Input: part model. Units: mm. Frame: model coordinates. Face numbers are marked on the shaded views. A direction names the side the tool comes from. Give positions to 0.01 mm unless a question says otherwise; leave off trailing zeros. Loops run counter-clockwise (first coordinate to the right, second up) from the corner with the lowest first, then second, coordinate; pieces in that order, holes last.
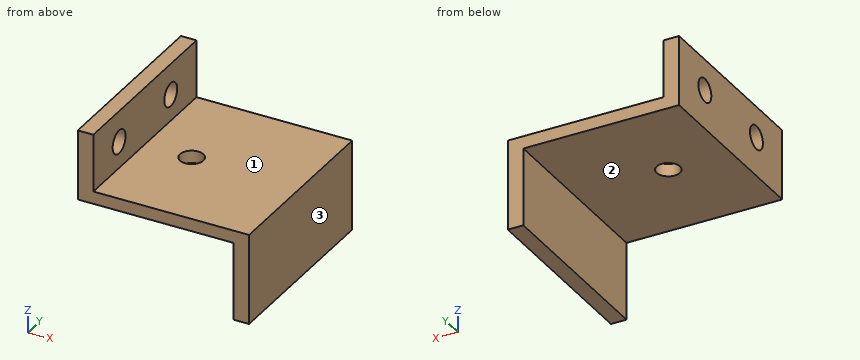
from build123d import *

# Parameters (mm, degrees)
RESSALTO_EXTRUS_O2_DEPTH = 24
ESBO_O2_R                = 1.5
CORTE_EXTRUS_O1_DEPTH    = 24
ESBO_O6_R                = 1.5
CORTE_EXTRUS_O2_DEPTH    = 13


with BuildPart() as part:
    # Esboço1 → Ressalto-extrusão2 (new body)
    with BuildSketch(Plane(origin=(0, 0, 0), x_dir=(1, 0, 0), z_dir=(0, 1, 0))):
        Polygon((0, 0), (0, -7.4), (2, -7.4), (2, 0), (22, 0), (22, 11.6), (20, 11.6), (20, 1.6), (0, 1.6), align=None)
    extrude(amount=RESSALTO_EXTRUS_O2_DEPTH)

    # Esboço2 → Corte-extrusão1 (cut)
    with BuildSketch(Plane.ZY):
        with Locations((3.4, 18)):
            Circle(ESBO_O2_R)
        with Locations((3.4, 6)):
            Circle(ESBO_O2_R)
    extrude(amount=-CORTE_EXTRUS_O1_DEPTH, mode=Mode.SUBTRACT)

    # Esboço6 → Corte-extrusão2 (cut)
    with BuildSketch(Plane(origin=(0, 0, -1.6), x_dir=(-1, 0, 0), z_dir=(0, 0, -1))):
        with Locations((-8, 12)):
            Circle(ESBO_O6_R)
    extrude(amount=-CORTE_EXTRUS_O2_DEPTH, mode=Mode.SUBTRACT)


solid = part.part
(1) Cut plane A-A (y = 12). Return the cut outline in (x, z).
Values follow:
outline: (0, -1.6) - (6.5, -1.6) - (6.5, 0) - (2, 0) - (2, 7.4) - (0, 7.4) - close; (9.5, -1.6) - (20, -1.6) - (20, -11.6) - (22, -11.6) - (22, 0) - (9.5, 0) - close
(2) Pin query (flat end, axial travel): pin 1 Ø2.5 at (x, y) = (8, 12) entering from -Z; pin 2 Ø4 at (x, y) = (17.5, 9) entering from +Z; pin 3 Ø6 at (x, y) = (4.5, 2.5) entering from -Z; pin 4 Ø11 at (y, z) = (10.5, -8.5) entering from -X. Return the tip coordinate at first contact, or that it passes through.
Values follow:
pin 1: passes through
pin 2: stops at z = 0
pin 3: stops at z = -1.6
pin 4: stops at x = 20
(3) Cut plane B-B (z = 3.4). Return the cut outline in (x, y).
Values follow:
outline: (0, 0) - (2, 0) - (2, 4.5) - (0, 4.5) - close; (0, 7.5) - (2, 7.5) - (2, 16.5) - (0, 16.5) - close; (0, 19.5) - (2, 19.5) - (2, 24) - (0, 24) - close
(4) Cut plane D-D (y = 18). Return the cut outline in (x, z), and give its area (3 significant figures).
Values follow:
outline: (0, -1.6) - (20, -1.6) - (20, -11.6) - (22, -11.6) - (22, 0) - (2, 0) - (2, 1.9) - (0, 1.9) - close; (0, 4.9) - (2, 4.9) - (2, 7.4) - (0, 7.4) - close
area: 64.0 mm2
(5) Cut plane C-C (x = 8). Return the cut outline in (y, z), and give its area (3 significant figures).
Values follow:
outline: (0, -1.6) - (10.5, -1.6) - (10.5, 0) - (0, 0) - close; (13.5, -1.6) - (24, -1.6) - (24, 0) - (13.5, 0) - close
area: 33.6 mm2
(6) Ray query, probe 1 along Y at (x, z) = (0.5, 3.4); probe 2 along Y at (x, z) = (8, -0.95); probe 3 along Z at (x, y) = (5.75, 7.75). Return the intervals inside material, ascending.
Values follow:
probe 1: y = 0 to 4.5, 7.5 to 16.5, 19.5 to 24
probe 2: y = 0 to 10.5, 13.5 to 24
probe 3: z = -1.6 to 0
(7) Reachability of the marked faces 1, 2 and 3 from +Z, -Z, +X, -X, +Y, -Y: full face, straight path, thin tool, end or side. Return the list, or none.
Values follow:
face 1: +Z, +X, +Y, -Y
face 2: -Z, -X, +Y, -Y
face 3: +Z, -Z, +X, +Y, -Y
